```python
from build123d import *

# Parameters (mm, degrees)
F0_R     = 6.15
F1_DEPTH = 30
F2_R     = 6
F3_SIZE2 = 0.57735
F3_SIZE  = 1


with BuildPart() as f1:
    # F0 (on Top) → F1 (new body)
    with BuildSketch(Plane.XY):
        Circle(F0_R)
    extrude(amount=F1_DEPTH)

    # F2
    f2_edges = [f1.edges().sort_by_distance(p)[0] for p in [
        (-6.15, 0, 30),
    ]]
    fillet(f2_edges, radius=F2_R)

    # F3
    f3_edges = [f1.edges().sort_by_distance(p)[0] for p in [
        (-6.15, 0, 0),
    ]]
    chamfer(f3_edges, length=F3_SIZE, length2=F3_SIZE2)


solid = f1.part
```
Could you check a few things on this model? Use its own coordinates, in mm. Round coordinates to 2 decimals unless told otherwise and drop trailing zeros. Loops run counter-clockwise (first coordinate to the right, second up) from the corner with the lowest first, then second, coordinate; pieces in that order, holes last.
Q1. For P1, Ø1.5, axis at x = -1.5, z = 22.5, coming from the +Y side; P2, Ø1.5, axis at x = -4, y = -0.5, coming from the +Z side; P3, Ø2, axis at y = -3.5, z = 8, coming from the -X side, each with a flat end and sliding along its axis, tell me the tip position at first contact or that it passes through.
Q2. Please list where these lines run through material, in increasing order: L1, parallel to X at y = 0.25, z = 9.5; L2, parallel to X at y = 4.5, z = 25.5.
Q3. I want a section at A-A (z = 13). Write out the boundary of the cut face in (x, y).
Answer below:
1. P1: stops at y = 6.1
1. P2: stops at z = 29.12
1. P3: stops at x = -5.62
2. L1: x = -6.14 to 6.14
2. L2: x = -3.91 to 3.91
3. outline: circle Ø12.3 at (0, 0)
